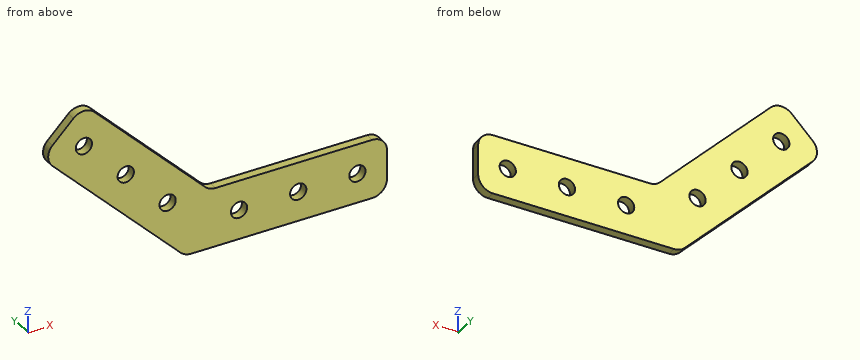
Autodesk Inventor part; units mm, degrees
ref_plane "YZ Plane" through (0, 0, 0) normal (1, 0, 0) x (0, 1, 0)
ref_plane "XZ Plane" through (0, 0, 0) normal (0, 1, 0) x (-1, 0, 0)
ref_plane "XY Plane" through (0, 0, 0) normal (0, 0, 1) x (1, 0, 0)
sketch "Skizze1" plane through (0, 0, 0) normal (0, 1, 0) x (-1, 0, 0)
  line L0 (-68.2843, 0) -> (0, 0)
  line L1 (0, 0) -> (48.2843, 48.2843)
  line L2 (48.2843, 48.2843) -> (34.1421, 62.4264)
  line L3 (34.1421, 62.4264) -> (-8.2843, 20)
  line L4 (-8.2843, 20) -> (-68.2843, 20)
  line L5 (-68.2843, 20) -> (-68.2843, 0)
  line L6 (-68.2843, 10) -> (-4.1421, 10) construction
  line L7 (-4.1421, 10) -> (41.2132, 55.3553) construction
  point P0 (-58.2843, 10)
  point P1 (-38.2843, 10)
  point P2 (-18.2843, 10)
  point P3 (5.8579, 20)
  point P4 (34.1421, 48.2843)
  point P5 (20, 34.1421)
  dimension "d3" = 60
  dimension "d4" = 20
  dimension "d5" = 135
  dimension "d6" = 10
  dimension "d7" = 30
  dimension "d8" = 50
  dimension "d9" = 10
  dimension "d10" = 30
  dimension "d11" = 50
extrude "Extrusion1" add sketch "Skizze1" along normal blind 3
fillet "Rundung1" radius 5 6 edges at (-34.1421, 1.5, 62.4264) (-48.2843, 1.5, 48.2843) (8.2843, 1.5, 20) (0, 1.5, 0) (68.2843, 1.5, 20) (68.2843, 1.5, 0)
hole "Bohrung1" at (58.2843, 0, 10) at (38.2843, 0, 10) at (18.2843, 0, 10) at (-5.8579, 0, 20) at (-34.1421, 0, 48.2843) at (-20, 0, 34.1421) direction (0, 1, 0) diameter 5.5 end through all
equation "\"d_tol\" = 0.3"
equation "\"d_wand\" = 1.5"
equation "\"D_oct\" = 3621.32034"
equation "\"d_traeger\" = 625"
equation "\"D_dode\" = 8196.15242"
equation "\"D_hexadeca\" = 7541.00924"
equation "\"r_rasp_pi\" = 3"
equation "\"b_rasp_pi\" = 56"
equation "\"l_rasp_pi\" = 85"
equation "\"w_kamera_vert\" = 41deg"
equation "\"w_kamera_hori\" = 66deg"
properties part number "Verbinder_45deg"
Model file for the job. Use its own axes, mm. Give positions to 0.01 mm unless a question says otherwise; leave off trailing zeros. Loops run counter-clockwise (first coordinate to the right, second up) from the corner with the lowest first, then second, coordinate; pieces in that order, holes last. Notation, with made-up numbers: (7, 71) -> (41, 71) arc R23 ccw to (41, 89) -> close; hole circle Ø4 at (54, 7). An arc over 180 degrees is marked (long way). Use CSV: the item, a comma, the result in double quotes. Start each with the question number.
1) Slice it at B-B on x = -20. Give the cut face in (y, z), plus the area to 3 significant figures.
2) Slice it at A-A on z = 10. Give the cut face in (x, y), plus the area to 3 significant figures.
3) Slice it at D-D on x = 43. Give the cut face in (y, z), plus the area to 3 significant figures.
4) Slice it at C-C on y = 2.3. Give the cut face in (x, z), plus the area to 3 significant figures.
5) Wall check: line 1 (X direction, y = 1.6, z = 10); line 2 (X direction, y = 1.3, z = 12.5); line 3 (Z direction, x = 14.5, y = 0.7). Give the ranges that are in metal, low to high.
6) Flat gauge pin, fed straight in: pin 1 Ø0.9 at (x, y) = (37, 2) entering from +Z. Where does the tip first touch, or does it go through?
Computed values:
1,outline,"(0, 20) -> (3, 20) -> (3, 31.39) -> (0, 31.39) -> close; (0, 36.89) -> (3, 36.89) -> (3, 48.28) -> (0, 48.28) -> close"
1,area,"68.4 mm^2"
2,outline,"(-10, 0) -> (15.53, 0) -> (15.53, 3) -> (-10, 3) -> close; (21.03, 0) -> (35.53, 0) -> (35.53, 3) -> (21.03, 3) -> close; (41.03, 0) -> (55.53, 0) -> (55.53, 3) -> (41.03, 3) -> close; (61.03, 0) -> (68.28, 0) -> (68.28, 3) -> (61.03, 3) -> close"
2,area,"185 mm^2"
3,outline,"(0, 0) -> (3, 0) -> (3, 20) -> (0, 20) -> close"
3,area,"60.0 mm^2"
4,outline,"(-44.75, 44.75) -> (-1.46, 1.46) arc R5 ccw to (2.07, 0) -> (63.28, 0) arc R5 ccw to (68.28, 5) -> (68.28, 15) arc R5 ccw to (63.28, 20) -> (10.36, 20) arc R5 cw to (6.82, 21.46) -> (-30.61, 58.89) arc R5 ccw to (-37.68, 58.89) -> (-44.75, 51.82) arc R5 ccw to start; hole circle Ø5.5 at (-34.14, 48.28); hole circle Ø5.5 at (-20, 34.14); hole circle Ø5.5 at (-5.86, 20); hole circle Ø5.5 at (18.28, 10); hole circle Ø5.5 at (38.28, 10); hole circle Ø5.5 at (58.28, 10)"
4,area,"2,400 mm^2"
5,line 1,"x = -10 to 15.53, 21.03 to 35.53, 41.03 to 55.53, 61.03 to 68.28"
5,line 2,"x = -12.5 to 17.14, 19.43 to 37.14, 39.43 to 57.14, 59.43 to 68.28"
5,line 3,"z = 0 to 20"
6,pin 1,"stops at z = 20"
